```python
from build123d import *

# Parameters (mm, degrees)
SKETCH1_R               = 3.1115
BOSS_EXTRUDE1_DEPTH     = 3.1496
SKETCH3_R               = 2.794
BOSS_EXTRUDE2_DEPTH     = 3.0988
SKETCH4_R               = 4.2291
BOSS_EXTRUDE3_DEPTH     = 3.81
CUT_EXTRUDE1_DEPTH      = 12.702221335
CUT_EXTRUDE1_DEPTH_BACK = 12.702221335
SKETCH5_R               = 1.4732
FILLET1_R               = 2.54


with BuildPart() as part:
    # Sketch1 → Boss-Extrude1 (new body)
    with BuildSketch(Plane(origin=(0, 0, 0), x_dir=(1, 0, 0), z_dir=(0, 1, 0))):
        with Locations(Location((0, 0, 0), (0, 0, 270))):
            Circle(SKETCH1_R)
    extrude(amount=BOSS_EXTRUDE1_DEPTH)

    # Sketch3 → Boss-Extrude2 (add)
    with BuildSketch(Plane(origin=(0, 3.1496, 0), x_dir=(1, 0, 0), z_dir=(0, 1, 0))):
        with Locations(Location((0, 0, 0), (0, 0, 270))):
            Circle(SKETCH3_R)
    extrude(amount=BOSS_EXTRUDE2_DEPTH)

    # Sketch4 → Boss-Extrude3 (add)
    with BuildSketch(Plane(origin=(0, 6.2484, 0), x_dir=(1, 0, 0), z_dir=(0, 1, 0))):
        with Locations(Location((0, 0, 0), (0, 0, 90))):
            Circle(SKETCH4_R)
    extrude(amount=BOSS_EXTRUDE3_DEPTH)

    # Sketch5 → Cut-Extrude1 (cut, two sides: drawn at the far end of the back side and taken through both)
    with BuildSketch(Plane(origin=(0, 10.0584, 0), x_dir=(1, 0, 0), z_dir=(0, 1, 0)).offset(-CUT_EXTRUDE1_DEPTH_BACK)):
        with Locations(Location((0, 0, 0), (0, 0, 270))):
            Circle(SKETCH5_R)
    extrude(amount=CUT_EXTRUDE1_DEPTH + CUT_EXTRUDE1_DEPTH_BACK, mode=Mode.SUBTRACT)

    # Fillet1
    fillet1_edges = [part.edges().sort_by_distance(p)[0] for p in [
        (0, 10.0584, 4.2291),
    ]]
    fillet(fillet1_edges, radius=FILLET1_R)


solid = part.part
```
Check sheet for the modelled part. Datum: model origin and axes. Units: mm. A direction names the side the tool comes from. Round coordinates to 2 decimals unless told otherwise and drop trailing zeros. Loops run counter-clockwise (first coordinate to the right, second up) from the corner with the lowest first, then second, coordinate; pieces in that order, holes last. Notation, with made-up numbers: (64, 76) -> (78, 76) arc R17 ccw to (78, 91) -> close; hole circle Ø4 at (88, 34). An arc over 180 degrees is marked (long way). Write item = value, one per line. Start each with the question number.
1) Release check for a two-part mould opening along Y. For faces 4 (the flat face through (3, 6.248, -1)), 5 (the cylindrical face through (-1.27, 6.875, -4.034)) record: released by +Y, released by -Y, zero draft, split by the parting line, or undercut.
2) Sectioned sample at B-B, the plane y = 0.5. Record the cut outline in (x, z), plus the area to 3 significant figures.
3) Set-up check for faces 1 (the cylindrical face through (-3.04, 1.55, -0.67)), 2 (the cylindrical face through (-2.728, 4.677, -0.606)), 3 (the cylindrical face through (1.46, 4.96, -0.19)): record each of +Z, -Z, +X, -X, +Y, -Y from which the full face is reachable in a straight line by a thin tool's end or side.
4) Gauge pin test, flat end, axial feed: pin 1 Ø5 at (x, y) = (-2.5, 1.5) entering from +Z. Record the tip position at first contact, or that the pin passes through.
5) Sectioned sample at A-A, the plane y = 7.25. Record the cut outline in (x, z), plus the area to 3 significant figures.
6) Thickness scan on probe 1 along X at (y, z) = (3, 0); probe 2 along X at (y, z) = (5.25, 0); probe 3 along Z at (x, y) = (1, 4.5). Record the ranges inside material, lowest first.
Results are:
q1.face_4 = undercut
q1.face_5 = zero draft
q2.outline = circle Ø6.22 at (0, 0); hole circle Ø2.95 at (0, 0)
q2.area = 23.6 mm^2
q3.face_1 = -Y
q3.face_2 = none
q3.face_3 = +Y, -Y
q4.pin_1 = 3.11
q5.outline = circle Ø8.46 at (0, 0); hole circle Ø2.95 at (0, 0)
q5.area = 49.4 mm^2
q6.probe_1 = -3.11 to -1.47, 1.47 to 3.11
q6.probe_2 = -2.79 to -1.47, 1.47 to 2.79
q6.probe_3 = -2.61 to -1.08, 1.08 to 2.61
